from build123d import *

# Parameters (mm, degrees)
SKETCH1_W               = 50
SKETCH1_H               = 50
SKETCH1_R               = 5
BOSS_EXTRUDE1_DEPTH     = 2.5
CUT_EXTRUDE2_DEPTH      = 36.707142143
CUT_EXTRUDE2_DEPTH_BACK = 5
FILLET1_R               = 1
CUT_EXTRUDE3_DEPTH      = 36.707142143


with BuildPart() as part:
    # Sketch1 → Boss-Extrude1 (new, symmetric)
    with BuildSketch(Plane.XY):
        Rectangle(SKETCH1_W, SKETCH1_H)
        Circle(SKETCH1_R, mode=Mode.SUBTRACT)
    extrude(amount=BOSS_EXTRUDE1_DEPTH, both=True)

    # Sketch4 → Cut-Extrude2 (cut, two sides: drawn at the far end of the back side and taken through both)
    with BuildSketch(Plane.XY.offset(2.5).offset(-CUT_EXTRUDE2_DEPTH_BACK)):
        Polygon((-5, 25), (-15, 25), (-15, 20), align=None)
    extrude(amount=CUT_EXTRUDE2_DEPTH + CUT_EXTRUDE2_DEPTH_BACK, mode=Mode.SUBTRACT)

    # Fillet1
    fillet1_edges = [part.edges().sort_by_distance(p)[0] for p in [
        (-15, 20, 0),
    ]]
    fillet(fillet1_edges, radius=FILLET1_R)

    # Sketch5 → Cut-Extrude3 (cut, through all)
    with BuildSketch(Plane.XY.offset(2.5)):
        with BuildLine():
            Line((-6.790302071, -10.325835977), (-14.674164023, -18.209697929))
            ThreePointArc((-14.674164023, -18.209697929), (-18.209697929, -18.209697929), (-18.209697929, -14.674164023))
            Line((-18.209697929, -14.674164023), (-10.325835977, -6.790302071))
            ThreePointArc((-10.325835977, -6.790302071), (-6.790302071, -6.790302071), (-6.790302071, -10.325835977))
        make_face()
    extrude(amount=-CUT_EXTRUDE3_DEPTH, mode=Mode.SUBTRACT)


solid = part.part
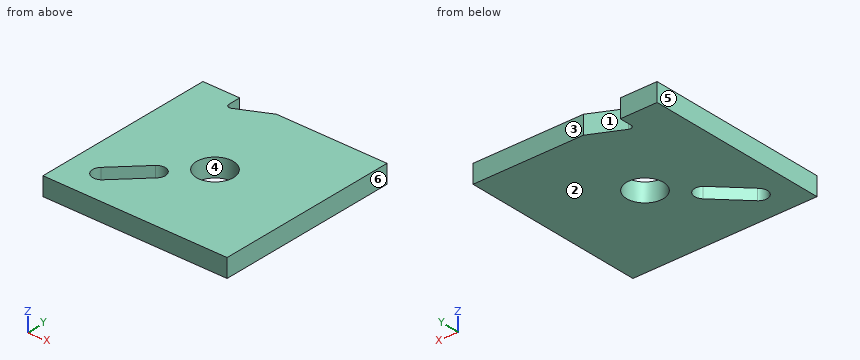
Source: CAD feature listing. Evaluate the final solid. Frame: model axes, mm. Face numbers are marked on the shaded views. A direction names the side the tool comes from. Round coordinates to 2 decimals unless told otherwise and drop trailing zeros. Write each loop counter-clockwise with the first axis right and the second up, starting at its lowest first coordinate (ties: lowest second). Pieces come first, ordered by that corner, then holes. Notation, with made-up numbers: (78.25, -8.5) - (84.25, -8.5) arc R16 cw to (84.25, 4.5) - close; hole circle Ø6 at (55, 17.25). An arc over 180 degrees is marked (long way). Use CSV: the item, a comma, the result in double quotes. Start each with the question number.
(1) Material intervals for probe 1 along Y at (x, z) = (0, -0.9); probe 2 along X at (y, z) = (-11, 0.35); probe 3 along X at (y, z) = (-2.5, 0.15), sorted ascending. Write a range as [from, to].
(2) Set-up query: the marked faces 1 and 2. Return all of +Z, -Z, +X, -X, +Y, -Y with unobstructed straight access to the full face (end or side cutting, diameter ignored); none if empty.
(3) Cut plane A-A, the plane y = 0. Return loops of the section in (x, z), and give its area (3 significant figures).
(4) Cut plane C-C, the plane z = 0.25. Return loops of the section in (x, y), and give its area (3 significant figures).
(5) Mould query, pull axis X, two halves, no side actions, for the marked faces 3, 4, 5 and 6. Classes: pulls with the +X half, pulls with the -X half, needs draft (parallel to the pull), parting line crosses it, or undercut.
Geometry says:
1,probe 1,"[-25, -5], [5, 25]"
1,probe 2,"[-25, -14.54], [-7.46, 25]"
1,probe 3,"[-25, -4.33], [4.33, 25]"
2,face 1,"+Z, -Z, +Y"
2,face 2,"-Z, +X, -X, +Y, -Y"
3,outline,"(-25, -2.5) - (-5, -2.5) - (-5, 2.5) - (-25, 2.5) - close; (5, -2.5) - (25, -2.5) - (25, 2.5) - (5, 2.5) - close"
3,area,"200 mm²"
4,outline,"(-25, -25) - (25, -25) - (25, 25) - (-5, 25) - (-13.55, 20.72) arc R1 cw to (-15, 21.62) - (-15, 25) - (-25, 25) - close; hole (-18.21, -14.67) arc R2.5 ccw to (-14.67, -18.21) - (-6.79, -10.33) arc R2.5 ccw to (-10.33, -6.79) - close; hole circle Ø10 at (0, 0)"
4,area,"2,320 mm²"
5,face 3,"needs draft"
5,face 4,"undercut"
5,face 5,"pulls with the -X half"
5,face 6,"pulls with the +X half"
